```python
from build123d import *

# Parameters (mm, degrees)
BOSS_EXTRUDE1_DEPTH = 16.002
FILLET1_R           = 1.27
SKETCH2_R           = 2.413
CUT_EXTRUDE1_DEPTH  = 40.990161384
SKETCH3_R           = 0.79375
CUT_EXTRUDE2_DEPTH  = 40.021802416


with BuildPart() as part:
    # Sketch1 → Boss-Extrude1 (new body)
    with BuildSketch(Plane(origin=(0, 0, 0), x_dir=(1, 0, 0), z_dir=(0, 1, 0))):
        Polygon((4.404264151, -0.835084906), (4.404264151, 9.578915094), (-26.329735849, 9.578915094), (-26.329735849, 4.816415094), (-16.804735849, 4.816415094), (-16.804735849, -0.835084906), align=None)
        Polygon((35.138264151, 4.816415094), (35.138264151, 9.578915094), (4.404264151, 9.578915094), (4.404264151, -0.835084906), (25.613264151, -0.835084906), (25.613264151, 4.816415094), align=None)
    extrude(amount=BOSS_EXTRUDE1_DEPTH)

    # Fillet1
    fillet1_edges = [part.edges().sort_by_distance(p)[0] for p in [
        (-16.804735849, 8.001, 0.835084906),
        (-16.804735849, 8.001, -4.816415094),
        (-26.329735849, 8.001, -4.816415094),
        (35.138264151, 8.001, -4.816415094),
        (25.613264151, 8.001, -4.816415094),
        (25.613264151, 8.001, 0.835084906),
    ]]
    fillet(fillet1_edges, radius=FILLET1_R)

    # Sketch2 → Cut-Extrude1 (cut, through all)
    with BuildSketch(Plane.XY.offset(0.835084906)):
        with Locations((4.404264151, 8.001)):
            Circle(SKETCH2_R)
    extrude(amount=-CUT_EXTRUDE1_DEPTH, mode=Mode.SUBTRACT)

    # Sketch3 → Cut-Extrude2 (cut, through all)
    with BuildSketch(Plane.XY.offset(-4.816415094)):
        with Locations((-21.567235849, 8.001)):
            Circle(SKETCH3_R)
        with Locations((30.375764151, 8.001)):
            Circle(SKETCH3_R)
    extrude(amount=-CUT_EXTRUDE2_DEPTH, mode=Mode.SUBTRACT)


solid = part.part
```
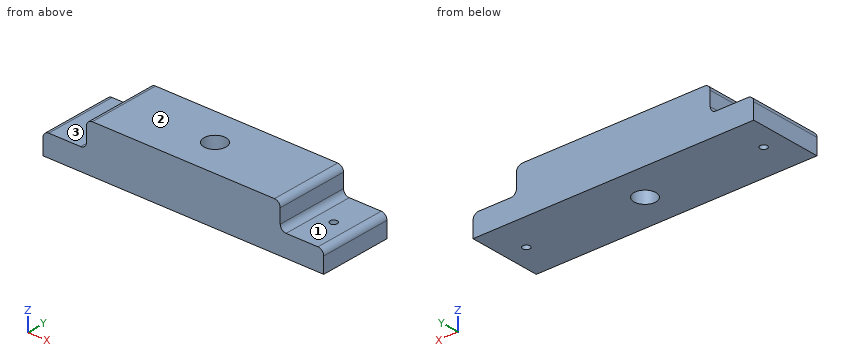
Input: part model. Units: mm. Frame: model coordinates. Face numbers are marked on the shaded views. A direction names the side the tool comes from. Give positions to 0.01 mm unless a question says otherwise; leave off trailing zeros. Write each loop counter-clockwise with the first axis right and the second up, starting at its lowest first coordinate (ties: lowest second). Pieces come first, ordered by that corner, then holes. Notation, with made-up numbers: (43, 40) - (88, 40) arc R15 ccw to (88, 64) - close; hole circle Ø11 at (-6.5, 84). An arc over 180 degrees is marked (long way). Write item = value, one per line. Start each with the question number.
1) Cut plane A-A (y = 13.75). Return loops of the section in (x, z), and give its area (3 significant figures).
2) Material intervals for L1, parallel to X at y = 7.75, z = -3.5; L2, parallel to Y at x = 30.5, z = -7.75; L3, parallel to Y at x = -22, z = -5.75, sorted ascending. Write a range as [from, to].
3) Reachability of the marked faces 1, 2 and 3 from +Z, -Z, +X, -X, +Y, -Y: full face, straight path, thin tool, end or side. Return the list, or none.
4) Pin query (flat end, axial travel): pin 1 (5 mm diameter, centred on y = 13.5, z = -1, fed in from +X); pin 2 (3.5 mm diameter, centred on x = -20.5, y = 5, fed in from +Z); pin 3 (7.5 mm diameter, centred on x = 30, y = 5.5, fed in from +Z); pin 4 (1.3 mm diameter, centred on x = 30.38, y = 8, fed in from -Z). Return the tip coordinate at first contact, or that it passes through.
5) Cut plane D-D (z = -1.25). Return loops of the section in (x, y).
6) Cut plane C-C (y = 6.5). Return loops of the section in (x, z).
7) Cut plane B-B (x = 4.5). Return loops of the section in (y, z).
Answers follow:
q1.outline = (-26.33, -9.58) - (35.14, -9.58) - (35.14, -6.09) arc R1.27 ccw to (33.87, -4.82) - (26.88, -4.82) arc R1.27 cw to (25.61, -3.55) - (25.61, -0.43) arc R1.27 ccw to (24.34, 0.84) - (-15.53, 0.84) arc R1.27 ccw to (-16.8, -0.43) - (-16.8, -3.55) arc R1.27 cw to (-18.07, -4.82) - (-25.06, -4.82) arc R1.27 ccw to (-26.33, -6.09) - close
q1.area = 532 mm^2
q2.L1 = [-16.8, 2], [6.8, 25.61]
q2.L2 = [0, 7.22], [8.78, 16]
q2.L3 = [0, 7.34], [8.67, 16]
q3.face_1 = +Z, +X, +Y, -Y
q3.face_2 = +Z, +X, -X, +Y, -Y
q3.face_3 = +Z, -X, +Y, -Y
q4.pin_1 = 25.61
q4.pin_2 = -4.82
q4.pin_3 = -4.65
q4.pin_4 = through
q5.outline = (-16.8, 0) - (25.61, 0) - (25.61, 16) - (-16.8, 16) - close; hole circle Ø4.83 at (4.4, 8)
q6.outline = (-26.33, -9.58) - (2.51, -9.58) - (2.51, 0.84) - (-15.53, 0.84) arc R1.27 ccw to (-16.8, -0.43) - (-16.8, -3.55) arc R1.27 cw to (-18.07, -4.82) - (-25.06, -4.82) arc R1.27 ccw to (-26.33, -6.09) - close; (6.29, -9.58) - (35.14, -9.58) - (35.14, -6.09) arc R1.27 ccw to (33.87, -4.82) - (26.88, -4.82) arc R1.27 cw to (25.61, -3.55) - (25.61, -0.43) arc R1.27 ccw to (24.34, 0.84) - (6.29, 0.84) - close
q7.outline = (0, -9.58) - (5.59, -9.58) - (5.59, 0.84) - (0, 0.84) - close; (10.41, -9.58) - (16, -9.58) - (16, 0.84) - (10.41, 0.84) - close
